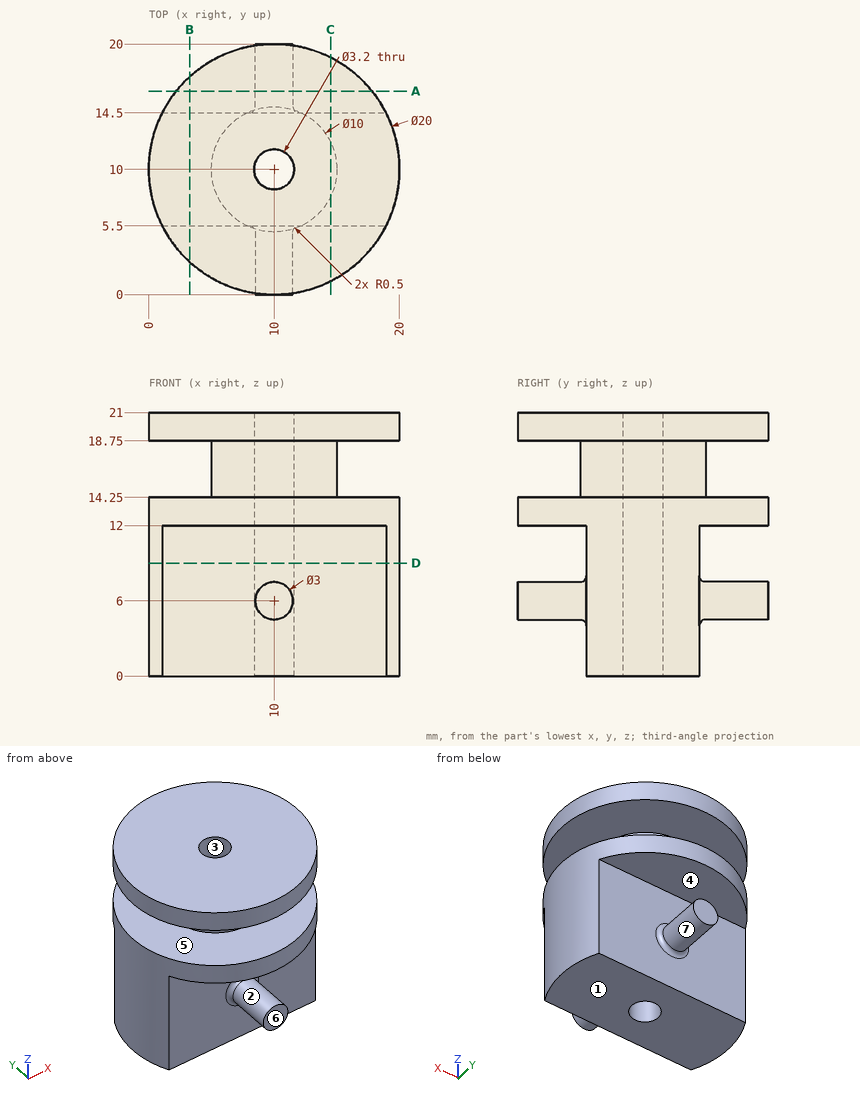
Can you work these out from the drawing? Everything is in mm from the part's minimum corner. A direction names the side the tool comes from. Coordinates: 2 decimals unless noted, no trailing zeros. Write each loop counter-clockwise with the first axis right and the second up, starting at its lowest first coordinate (ties: lowest second). Pieces come first, ordered by that corner, then holes. Notation, with made-up numbers: (-29, 59) - (-19, 59) arc R31 ccw to (-19, 90) - close; hole circle Ø11 at (-9, 5). An arc over 180 degrees is marked (long way). Use a Markdown table: item, result.
Q1. Thinking about a two-plate mould opening in Z: for the marked faces 1, 2 and 3, which applies, +Z half, -Z half, draft (parallel to the pull), parting line (faces both ways), or undercut?
Geometry check:
| item | result |
|---|---|
| face 1 | -Z half |
| face 2 | undercut |
| face 3 | draft |
Q2. Please list where these lines run through material, in increasing order: L1, parallel to Z at x = 3.75, y = 8.25; L2, parallel to Z at x = 8, y = 1.75; L3, parallel to Y at x = 1.5, z = 5.
Geometry check:
| item | result |
|---|---|
| L1 | z = 0 to 14.25, 18.75 to 21 |
| L2 | z = 12 to 14.25, 18.75 to 21 |
| L3 | y = 5.5 to 14.5 |
Q3. I'm going to push flat-ended pins straight in: pin 1 Ø3.5 at (x, z) = (6, 8.5) entering from +Y; pin 2 Ø1.5 at (y, z) = (3, 7.5) entering from -X; pin 3 Ø4.5 at (x, y) = (9.5, 18.5) entering from -Z. Where does each tip first touch, or does it pass through?
Geometry check:
| item | result |
|---|---|
| pin 1 | stops at y = 14.5 |
| pin 2 | stops at x = 8.7 |
| pin 3 | stops at z = 4.5 |
Q4. Imagine slicing it at A-A (y = 16.25). List the corners of the cut face in (x, z) for me.
Geometry check:
| item | result |
|---|---|
| outline | (2.19, 12) - (17.81, 12) - (17.81, 14.25) - (2.19, 14.25) - close; (2.19, 18.75) - (17.81, 18.75) - (17.81, 21) - (2.19, 21) - close; circle Ø3 at (10, 6) |
Q5. Imagine slicing it at C-C (x = 14.5). List the corners of the cut face in (y, z) for me.
Geometry check:
| item | result |
|---|---|
| outline | (1.07, 12) - (5.5, 12) - (5.5, 0) - (14.5, 0) - (14.5, 12) - (18.93, 12) - (18.93, 14.25) - (12.18, 14.25) - (12.18, 18.75) - (18.93, 18.75) - (18.93, 21) - (1.07, 21) - (1.07, 18.75) - (7.82, 18.75) - (7.82, 14.25) - (1.07, 14.25) - close |
Q6. Which directions (+Z, -Z, +X, -X, +Y, -Y) give clear straight access to the entire face, cutting with the end or side of a thin tool? Please do the marked faces 4, 5, 6 and 7.
Geometry check:
| item | result |
|---|---|
| face 4 | +X, -X, +Y |
| face 5 | none |
| face 6 | +Z, -Z, +X, -X, -Y |
| face 7 | +Y |
Q7. Imagine slicing it at D-D (z = 9). List the corners of the cut face in (x, y) for me, and give its area (3 significant figures).
Geometry check:
| item | result |
|---|---|
| outline | (1.07, 5.5) - (18.93, 5.5) arc R10 ccw to (18.93, 14.5) - (1.07, 14.5) arc R10 ccw to start; hole circle Ø3.2 at (10, 10) |
| area | 166 mm2 |
Q8. Imagine slicing it at B-B (x = 3.25). List the corners of the cut face in (y, z) for me, and give its area (3 significant figures).
Geometry check:
| item | result |
|---|---|
| outline | (2.62, 12) - (5.5, 12) - (5.5, 0) - (14.5, 0) - (14.5, 12) - (17.38, 12) - (17.38, 14.25) - (2.62, 14.25) - close; (2.62, 18.75) - (17.38, 18.75) - (17.38, 21) - (2.62, 21) - close |
| area | 174 mm2 |
